The drawing under review shows one solid part. Ordinate dimensions are in mm from its lowest x, y, z. A direction names the side the tool comes from. Round coordinates to 2 decimals unless told otherwise and drop trailing zeros. Write each loop counter-clockwise with the first axis right and the second up, starting at its lowest first coordinate (ties: lowest second). Pieces come first, ordered by that corner, then holes. Notation, with made-up numbers: M -10.75,-3 L 16.25,-3 A24 ccw 16.25,19 Z; hole C -1,83.25 d7. An arc over 180 degrees is marked long. Write item = value, one per line. Start each with the question number.
Item 1: For pin 1 Ø3 at (x, y) = (29, 3) entering from -Z; pin 2 Ø15 at (x, z) = (13.5, 395) entering from -Y (3 decimals); pin 3 Ø7.5 at (x, y) = (16.5, 3.5) entering from +Z, all flat-tipped, find the tip position at first contact; note any pin that passes through.
Item 2: Tool access review of the marked faces 1 and 2: name each direction out of +Z, -Z, +X, -X, +Y, -Y from which nothing blocks a thin tool from reaching the whole face with its end or side.
Item 3: Take a section at B-B, the plane x = 11.5. Give the boundary of the cut face in (y, z) (3 decimals), plus the area to 3 significant figures.
Item 4: To check wall thickness, follow line 1 along Z through (x, y) = (2, 3.75); line 2 along Y through (x, z) = (12, 39) (3 decimals). State the ranges of each line that lie inside material, in increasing order.
Item 5: Take a section at A-A, the plane y = 6.5. Give the boundary of the cut face in (x, z).
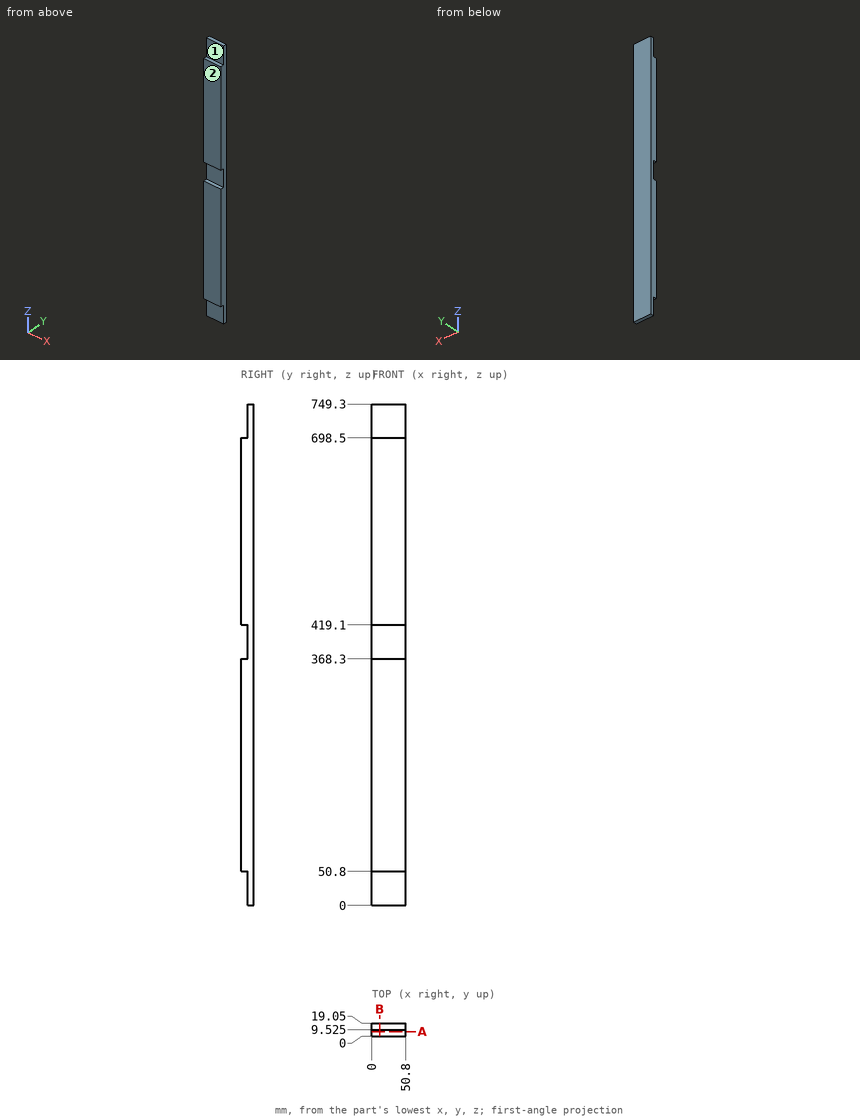
Response values:
q1.pin_1 = 50.8
q1.pin_2 = 9.525
q1.pin_3 = 698.5
q2.face_1 = +Z, +X, -X, -Y
q2.face_2 = +Z, -Z, +X, -X, -Y
q3.outline = M 0,50.8 L 9.525,50.8 L 9.525,0 L 19.05,0 L 19.05,749.3 L 9.525,749.3 L 9.525,698.5 L 0,698.5 L 0,419.1 L 9.525,419.1 L 9.525,368.3 L 0,368.3 Z
q3.area = 12,800 mm2
q4.line_1 = 50.8 to 368.3, 419.1 to 698.5
q4.line_2 = 9.525 to 19.05
q5.outline = M 0,50.8 L 50.8,50.8 L 50.8,368.3 L 0,368.3 Z; M 0,419.1 L 50.8,419.1 L 50.8,698.5 L 0,698.5 Z
